Read the model definition and answer for the solid it produces. Units are mm, in the model's axes. Face numbers are marked on the shaded views. A direction names the side the tool comes from. Round coordinates to 2 decimals unless told otherwise and drop trailing zeros. Loops run counter-clockwise (first coordinate to the right, second up) from the corner with the lowest first, then second, coordinate; pieces in that order, holes last. Notation, with made-up numbers: M -26,-15.75 L -17,-15.75 A33 ccw -17,22.25 Z; hole C 6.25,78.5 d7. An arc over 180 degrees is marked long. Write each question's results on one line, items separated by ' | '.
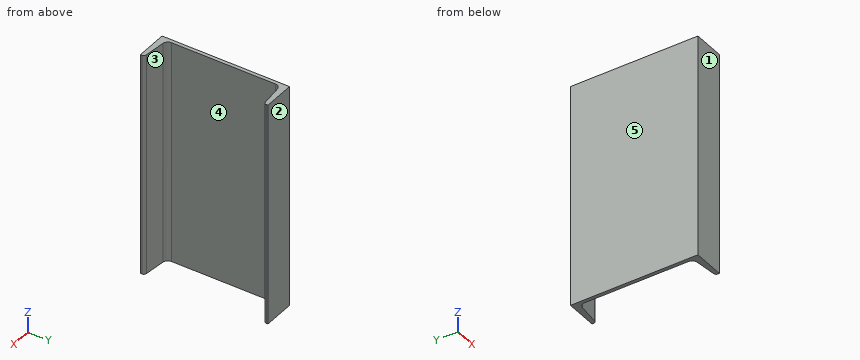
from build123d import *

# Parameters (mm, degrees)
BASEMCHANNEL_START = -350
BASEMCHANNEL_DEPTH = 700
TOEFILLET_R        = 8.5


# Read off the part's stored shape, not the designer's step: BaseMchannel
with BuildPart() as part:
    # BaseMchannel outline → BaseMchannel (new body)
    with BuildSketch(Plane.XY.offset(BASEMCHANNEL_START)):
        with BuildLine():
            Line((0, 400), (0, 0))
            Line((0, 0), (100, 0))
            Line((100, 0), (100, 12.322861527))
            Line((100, 12.322861527), (26.223016124, 20.077134998))
            ThreePointArc((26.223016124, 20.077134998), (15.366537967, 25.608786911), (11, 36.984007219))
            Line((11, 36.984007219), (11, 363.015992781))
            ThreePointArc((11, 363.015992781), (15.366537967, 374.391213089), (26.223016124, 379.922865002))
            Line((26.223016124, 379.922865002), (100, 387.677138473))
            Line((100, 387.677138473), (100, 400))
            Line((100, 400), (0, 400))
        make_face()
    extrude(amount=BASEMCHANNEL_DEPTH)

    # ToeFillet
    toefillet_edges = [part.edges().sort_by_distance(p)[0] for p in [
        (100, 387.677138473, 0),
        (100, 12.322861527, 0),
    ]]
    fillet(toefillet_edges, radius=TOEFILLET_R)


solid = part.part
Item 1: The mould has two halves that part along Y. Classify the marked faces 1, 2 and 3: pulls with the +Y half, pulls with the -Y half, needs draft (parallel to the pull), parting line crosses it, or undercut.
Outcome:
face 1: pulls with the -Y half | face 2: pulls with the +Y half | face 3: undercut
Item 2: The part is cut by section B-B (z = 187.5). Determine the outline of the cut face in (x, y), plus the area to 3 significant figures.
Outcome:
outline: M 0,0 L 100,0 L 100,4.67 A8.5 ccw 92.39,13.12 L 26.22,20.08 A17 cw 11,36.98 L 11,363.02 A17 cw 26.22,379.92 L 92.39,386.88 A8.5 ccw 100,395.33 L 100,400 L 0,400 Z | area: 7,500 mm2
Item 3: Straight lines are drawn through the part: line 1 (Y direction, x = 26, z = -155); line 2 (Y direction, x = 90, z = 52); line 3 (X direction, y = 64, z = 210). For each, find the intervals that lie inside material, in ascending order.
Outcome:
line 1: y = 0 to 20.1, 379.9 to 400 | line 2: y = 0 to 13.37, 386.63 to 400 | line 3: x = 0 to 11
Item 4: The part is cut by section A-A (x = 84). Determine the outline of the cut face in (y, z).
Outcome:
outline: M 0,-350 L 14,-350 L 14,350 L 0,350 Z; M 386,-350 L 400,-350 L 400,350 L 386,350 Z
Item 5: A flat-ended cylindrical pin translates along its axis: pin 1 (4 mm diameter, centred on y = 255, z = -164.5, fed in from +X). Find the tip coordinate at first contact, or state that the pin passes through.
Outcome:
pin 1: stops at x = 11
Item 6: The part is cut by section C-C (y = 352). Determine the outline of the cut face in (x, z), plus the area to 3 significant figures.
Outcome:
outline: M 0,-350 L 11,-350 L 11,350 L 0,350 Z | area: 7,700 mm2
Item 7: The part is cut by section D-D (x = 46.5). Determine the outline of the cut face in (y, z).
Outcome:
outline: M 0,-350 L 17.95,-350 L 17.95,350 L 0,350 Z; M 382.05,-350 L 400,-350 L 400,350 L 382.05,350 Z
Item 8: For the marked faces 4 and 5, determine the directions among +Z, -Z, +X, -X, +Y, -Y from which every point of the face is accessible in a straight line to the end or side of a thin tool.
Outcome:
face 4: +Z, -Z, +X | face 5: +Z, -Z, -X, +Y, -Y
